Part model, mm, in its own coordinate system. A direction names the side the tool comes from. Round coordinates to 2 decimals unless told otherwise and drop trailing zeros. Write each loop counter-clockwise with the first axis right and the second up, starting at its lowest first coordinate (ties: lowest second). Pieces come first, ordered by that corner, then holes. Notation, with made-up numbers: (5, 30.5) -> (25, 30.5) arc R13 ccw to (25, 49.5) -> close; hole circle Ø9 at (80.25, 76.5). An arc over 180 degrees is marked (long way). Use CSV: the item, a comma, the result in double quotes. Start each with the question number.
Autodesk Fusion 360 part; units mm, degrees
sketch "Esboço1" plane through (0, 0, 0) normal (0, 0, 1) x (1, 0, 0)
  line L0 (85, -70) -> (-85, -70)
  line L1 (-85, -70) -> (-85, 70)
  line L2 (-85, 70) -> (85, 70)
  line L3 (85, 70) -> (85, -70)
  line L4 (85, -70) -> (-85, 70) construction
  line L5 (-85, -70) -> (85, 70) construction
  dimension "d1" = 170
  dimension "d2" = 140
extrude "Extrusão1" add sketch "Esboço1" along normal blind 35
sketch "Esboço2" plane through (0, 0, 35) normal (0, 0, 1) x (-1, 0, 0)
  line L0 (-85, -70) -> (85, -70)
  line L1 (85, -70) -> (85, 70)
  line L2 (85, 70) -> (-85, 70)
  line L3 (-85, 70) -> (-85, -70)
  line L4 (-81, 66) -> (81, 66)
  line L5 (81, 66) -> (81, -66)
  line L6 (81, -66) -> (-81, -66)
  line L7 (-81, -66) -> (-81, 66)
  line L8 (-81, 66) -> (81, -66) construction
  line L9 (81, 66) -> (-81, -66) construction
  dimension "d5" = 162
  dimension "d6" = 132
extrude "Extrusão2" cut sketch "Esboço2" against normal blind 30 contours L4 L5 L6 L7
fillet "Arredondamento1" radius 3 4 edges at (-85, 70, 17.5) (-85, -70, 17.5) (85, -70, 17.5) (85, 70, 17.5)
1. Which spindle directions (+Z, -Z, +X, -X, +Y, -Y) get a long thin tool onto all of the face, cutting with end or side? Do faces 4 (the flat face through (1, -1, 5)), 5 (the flat face through (1, -70, 17)). Say none if no direction does.
2. Flat gauge pin, fed straight in: pin 1 (2 mm diameter, centred on x = 67.5, y = 11, fed in from +Z). Where does the tip first touch, or does it go through?
3. Drill centre lines: line 1 along X through (y, z) = (-24, 10); line 2 along Y through (x, z) = (-30, 30); line 3 along Z through (x, y) = (72.5, -57.5). Where is each one in solid material? Low to high. Write a range as [from, to].
4. Band-saw the part on B-B (x = 36). List the corners of the cut face in (y, z), then the cut area to 3 significant figures.
5. Band-saw the part on C-C (y = 30). List the corners of the cut face in (x, z), then the cut area to 3 significant figures.
6. Band-saw the part on A-A (z = 25). List the corners of the cut face in (x, y).
7. Pull direction Y, two halves, no side cores. Call faces 1 (the flat face through (-1, 70, 17)), 2 (the flat face through (-85, -1, 17)), 3 (the flat face through (81, 1, 20)): released by +Y, released by -Y, zero draft, split by the parting line, or undercut.
Answers below:
1,face 4,"+Z"
1,face 5,"+Z, -Z, +X, -X, -Y"
2,pin 1,"stops at z = 5"
3,line 1,"x = [-85, -81], [81, 85]"
3,line 2,"y = [-70, -66], [66, 70]"
3,line 3,"z = [0, 5]"
4,outline,"(-70, 0) -> (70, 0) -> (70, 35) -> (66, 35) -> (66, 5) -> (-66, 5) -> (-66, 35) -> (-70, 35) -> close"
4,area,"940 mm^2"
5,outline,"(-85, 0) -> (85, 0) -> (85, 35) -> (81, 35) -> (81, 5) -> (-81, 5) -> (-81, 35) -> (-85, 35) -> close"
5,area,"1,090 mm^2"
6,outline,"(-85, -67) arc R3 ccw to (-82, -70) -> (82, -70) arc R3 ccw to (85, -67) -> (85, 67) arc R3 ccw to (82, 70) -> (-82, 70) arc R3 ccw to (-85, 67) -> close; hole (-81, -66) -> (81, -66) -> (81, 66) -> (-81, 66) -> close"
7,face 1,"released by +Y"
7,face 2,"zero draft"
7,face 3,"undercut"
